The model under review builds one solid part; all positions refer to its coordinate system, in mm. Face numbers are marked on the shaded views. A direction names the side the tool comes from. Round coordinates to 2 decimals unless told otherwise and drop trailing zeros. Order: outer loops, then holes, each group sorted by start corner. A loop starts at its lowest first (then second) coordinate and runs counter-clockwise, first axis right, second up.
1) To check wall thickness, follow L1, parallel to X at y = 19.25, z = 12.5; L2, parallel to X at y = 32, z = -22; L3, parallel to X at y = 14.5, z = 21. State the ranges of each line that lie inside material, in increasing order.
2) Consider section A-A (y = 54.5). Give the boundary of the cut face in (x, z), then the cut area to 3 significant figures.
3) Mouldability with a two-part tool opening along X and no side actions: class the marked faces 1, 2, 3 and 4 as pulls with the +X half, pulls with the -X half, needs draft (parallel to the pull), parting line crosses it, or undercut.
4) Consider section D-D (y = 32.5). Give the boundary of the cut face in (x, z).
5) Clearance check with flat-ended pins moving along their axes: P1, Ø1.5, axis at x = -56, z = 4, coming from the +Y side; P2, Ø12, axis at x = -80, z = -8, coming from the -Y side; P3, Ø12.5, axis at y = 36.5, z = 16, coming from the +X side. State where each tip first meets the part, or that it passes through.
6) Consider section B-B (x = 86.7). Give the boundary of the cut face in (y, z).
7) Consider section C-C (z = -4.5). Give the boundary of the cut face in (x, y).
8) Machinability: for the marked faces 5, 6, 7, 8 and 9, which of the approach directions +Z, -Z, +X, -X, +Y, -Y give a long, thin tool a straight path to every point of the face, cutting with its end or side? Answer none if there is none.
from build123d import *

# Parameters (mm, degrees)
BOSS_EXTRUDE1_DEPTH = 25
SKETCH2_R           = 8
CUT_EXTRUDE1_DEPTH  = 70.5
SKETCH3_R           = 8
CUT_EXTRUDE2_DEPTH  = 88
SKETCH4_W           = 40
SKETCH4_H           = 25
BOSS_EXTRUDE2_DEPTH = 24.6
SKETCH5_R           = 7.5
CUT_EXTRUDE4_DEPTH  = 4.5
SKETCH7_W           = 25
SKETCH7_H           = 25
CUT_EXTRUDE6_DEPTH  = 20
SKETCH10_W          = 25
SKETCH10_H          = 12.5
CUT_EXTRUDE7_DEPTH  = 25
SKETCH13_W          = 12.503220776
SKETCH13_H          = 18.75
CUT_EXTRUDE9_DEPTH  = 25
SKETCH17_W          = 25
SKETCH17_H          = 25.299748734
CUT_EXTRUDE11_DEPTH = 8


with BuildPart() as part:
    # Sketch1 → Boss-Extrude1 (new body)
    with BuildSketch(Plane.XY):
        Polygon((59.2, 45), (-60.8, 45), (-60.8, 57.5), (-100.8, 57.5), (-100.8, 45), (-100.8, 20), (-100.8, 7.5), (-60.8, 7.5), (-60.8, 20), (59.2, 20), (59.2, 7.5), (99.2, 7.5), (99.2, 20), (74.2, 20), (74.2, 45), (99.2, 45), (99.2, 57.5), (59.2, 57.5), align=None)
    extrude(amount=BOSS_EXTRUDE1_DEPTH)

    # Sketch2 → Cut-Extrude1 (cut)
    with BuildSketch(Plane(origin=(0, 57.5, 0), x_dir=(1, 0, 0), z_dir=(0, 1, 0))):
        with Locations(Location((-88.3, -12.5, 0), (0, 0, 180))):
            Circle(SKETCH2_R)
    extrude(amount=-CUT_EXTRUDE1_DEPTH, mode=Mode.SUBTRACT)

    # Sketch3 → Cut-Extrude2 (cut)
    with BuildSketch(Plane(origin=(0, 57.5, 0), x_dir=(1, 0, 0), z_dir=(0, 1, 0))):
        with Locations(Location((86.7, -12.5, 0), (0, 0, 270))):
            Circle(SKETCH3_R)
    extrude(amount=-CUT_EXTRUDE2_DEPTH, mode=Mode.SUBTRACT)

    # Sketch4 → Boss-Extrude2 (add)
    with BuildSketch(Plane(origin=(0, 0, 0), x_dir=(-1, 0, 0), z_dir=(0, 0, -1))):
        with Locations((80.8, 32.5)):
            Rectangle(SKETCH4_W, SKETCH4_H)
    extrude(amount=BOSS_EXTRUDE2_DEPTH)

    # Sketch5 → Cut-Extrude4 (cut)
    with BuildSketch(Plane(origin=(0, 0, -24.6), x_dir=(-1, 0, 0), z_dir=(0, 0, -1))):
        with Locations((85.8, 32.5)):
            Circle(SKETCH5_R)
    extrude(amount=-CUT_EXTRUDE4_DEPTH, mode=Mode.SUBTRACT)

    # Sketch7 → Cut-Extrude6 (cut)
    with BuildSketch(Plane.XY.offset(25)):
        with Locations((-88.3, 32.5)):
            Rectangle(SKETCH7_W, SKETCH7_H)
    extrude(amount=-CUT_EXTRUDE6_DEPTH, mode=Mode.SUBTRACT)

    # Sketch10 → Cut-Extrude7 (cut)
    with BuildSketch(Plane.ZY.offset(100.8)):
        with Locations((0, 32.5)):
            Rectangle(SKETCH10_W, SKETCH10_H)
    extrude(amount=-CUT_EXTRUDE7_DEPTH, mode=Mode.SUBTRACT)

    # Sketch13 → Cut-Extrude9 (cut)
    with BuildSketch(Plane.XY.offset(25)):
        Polygon((-88.295569288, 41.830666142), (-88.296779224, 32.455666142), (-88.296779224, 23.080666142), (-75.8, 23.080666142), (-75.8, 41.830666142), align=None)
        with Locations((-69.548389612, 32.455666142)):
            Rectangle(SKETCH13_W, SKETCH13_H)
    extrude(amount=-CUT_EXTRUDE9_DEPTH, mode=Mode.SUBTRACT)

    # Sketch17 → Cut-Extrude11 (cut)
    with BuildSketch(Plane(origin=(74.2, 0, 0), x_dir=(0, 0, -1), z_dir=(1, 0, 0))):
        with Locations((-12.5, 32.350125633)):
            Rectangle(SKETCH17_W, SKETCH17_H)
    extrude(amount=-CUT_EXTRUDE11_DEPTH, mode=Mode.SUBTRACT)


solid = part.part
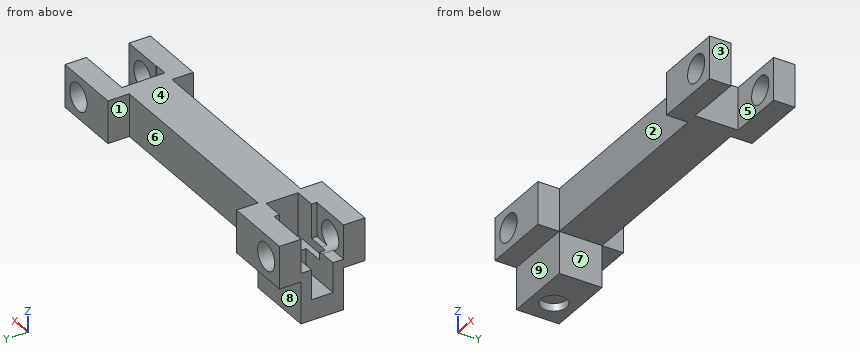
Answer below:
1. L1: x = -100.8 to -96.3, -80.3 to -60.8, 59.2 to 78.7, 94.7 to 99.2
1. L2: x = -100.8 to -93.28, -78.32 to -60.8
1. L3: x = -100.8 to -60.8, 59.2 to 99.2
2. outline: (-100.8, 0) - (-60.8, 0) - (-60.8, 25) - (-100.8, 25) - close; (59.2, 0) - (99.2, 0) - (99.2, 25) - (59.2, 25) - close; hole circle Ø16 at (-88.3, 12.5); hole circle Ø16 at (86.7, 12.5)
2. area: 1,600 mm2
3. face 1: undercut
3. face 2: undercut
3. face 3: pulls with the +X half
3. face 4: needs draft
4. outline: (-100.8, -24.6) - (-93.3, -24.6) - (-93.3, -20.1) - (-78.3, -20.1) - (-78.3, -24.6) - (-60.8, -24.6) - (-60.8, 0) - (66.2, 0) - (66.2, 25) - (-63.3, 25) - (-63.3, 0) - (-75.8, 0) - (-75.8, -12.5) - (-100.8, -12.5) - close
5. P1: stops at y = 45
5. P2: stops at y = 20
5. P3: stops at x = 66.2
6. outline: (7.5, 0) - (20, 0) - (20, 4.5) - (7.5, 4.5) - close; (7.5, 20.5) - (20, 20.5) - (20, 25) - (7.5, 25) - close; (45, 0) - (57.5, 0) - (57.5, 4.5) - (45, 4.5) - close; (45, 20.5) - (57.5, 20.5) - (57.5, 25) - (45, 25) - close
7. outline: (-100.8, 20) - (-60.8, 20) - (-60.8, 45) - (-100.8, 45) - (-100.8, 38.75) - (-75.8, 38.75) - (-75.8, 26.25) - (-100.8, 26.25) - close
8. face 5: +Z, -Z, +X
8. face 6: +Z, -Z, +Y
8. face 7: -Z, +X, +Y, -Y
8. face 8: -Z, +X, -X, +Y
8. face 9: -Z, +X, -X, -Y
